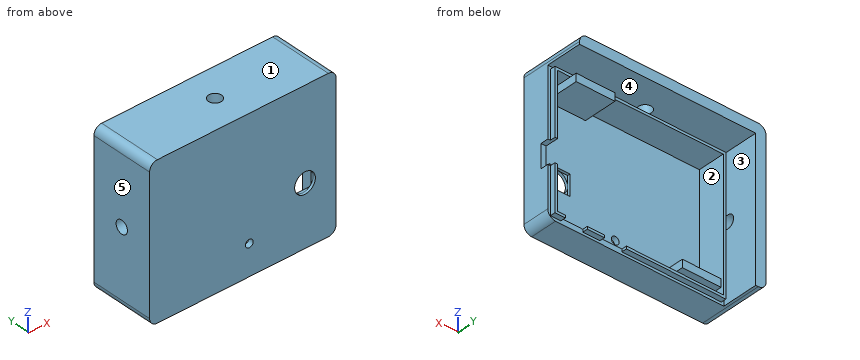
Autodesk Inventor part; units mm, degrees
ref_plane "YZ Plane" through (0, 0, 0) normal (1, 0, 0) x (0, 1, 0)
ref_plane "XZ Plane" through (0, 0, 0) normal (0, 1, 0) x (-1, 0, 0)
ref_plane "XY Plane" through (0, 0, 0) normal (0, 0, 1) x (1, 0, 0)
sketch "Sketch1" plane through (0, 0, 0) normal (0, 1, 0) x (-1, 0, 0)
  point P0 (0, 0)
sketch "Sketch2" plane through (0, 0, 0) normal (0, 1, 0) x (-1, 0, 0)
  line L0 (68, -12) -> (68, -66)
  line L1 (68, -66) -> (0, -66)
  line L2 (0, -66) -> (0, -12)
  line L3 (68, -12) -> (0, -12)
  point P0 (0, 0)
  dimension "d0" = 68
  dimension "d138" = 54
extrude "Extrusion1" add sketch "Sketch2" along normal blind 12.5
sketch "Sketch3" plane through (0, 12.5, 0) normal (0, 1, 0) x (1, 0, 0)
  point P0 (-68, 66)
sketch "Sketch4" plane through (0, 12.5, 0) normal (0, 1, 0) x (1, 0, 0)
  line L0 (0, 66) -> (-68, 66)
  line L1 (-30.4814, 66) -> (-28.4814, 66)
  line L2 (-28.4814, 66) -> (-28.4814, 64)
  line L3 (-68, 66) -> (-68, 12)
  line L4 (-68, 37.8423) -> (-68, 39.8423)
  line L5 (-68, 39.8423) -> (-66, 39.8423)
  line L6 (0, 38.8423) -> (0, 36.8423)
  line L7 (0, 36.8423) -> (-2, 36.8423)
  line L8 (-66, 64) -> (-2, 64)
  line L9 (-2, 64) -> (-2, 14)
  line L10 (-2, 14) -> (-66, 14)
  line L11 (-66, 14) -> (-66, 64)
  dimension "d5" = 2
  dimension "d6" = 2
  dimension "d7" = 2
  dimension "d11" = 2
  dimension "d75" = 2
  dimension "d132" = 50
  dimension "d133" = 64
extrude "Extrusion2" cut sketch "Sketch4" against normal blind 10.5 contours L8 L9 L10 L11
sketch "Sketch7" plane through (0, 12.5, 0) normal (0, 1, 0) x (1, 0, 0)
  line L0 (-68, 66) -> (-67, 66)
  line L1 (-68, 66) -> (-6, 66)
  line L2 (-68, 65) -> (-68, 66)
  line L3 (0, 66) -> (-7, 66)
  line L4 (-67, 65) -> (-1, 65)
  line L5 (0, 66) -> (-68, 66)
  line L6 (-68, 66) -> (0, 66)
  line L7 (0, 12) -> (0, 66)
  line L8 (0, 12) -> (-1, 12)
  line L9 (-1, 66) -> (0, 66)
  line L10 (0, 66) -> (0, 12)
  line L11 (0, 12) -> (-1, 12)
  line L12 (-68, 12) -> (0, 12)
  line L13 (-1, 65) -> (-1, 12)
  line L14 (0, 12) -> (-1, 12)
  line L15 (-67, 65) -> (-67, 12)
  line L16 (-68, 66) -> (-68, 12)
  line L17 (-67, 12) -> (-68, 12)
  line L18 (-68, 12) -> (-68, 66)
  dimension "d76" = 1
  dimension "d139" = 1
  dimension "d140" = 1
extrude "Extrusion3" cut sketch "Sketch7" against normal blind 2 contours L0 L1 L3 L7 L8 L13 L4 L15 L12 L16 L2
sketch "Sketch8" plane through (0, 12.5, 0) normal (0, 1, 0) x (1, 0, 0)
  line L0 (0, 12) -> (0, 13)
  line L1 (0, 13) -> (-68, 13)
  line L2 (0, 12) -> (-68, 12)
  line L3 (-68, 12) -> (-68, 13)
  line L4 (-67, 12) -> (-1, 12)
  point P0 (0, 0)
  point P1 (-70, 0)
  dimension "d46" = 68
  dimension "d141" = 1
extrude "Extrusion4" cut sketch "Sketch8" against normal blind 2
sketch "Sketch10" plane through (0, 2, 0) normal (0, 1, 0) x (1, 0, 0)
  line L0 (-31, 2) -> (-41, 2)
  line L1 (-63, 64) -> (-48, 64)
  line L2 (-48, 64) -> (-48, 61)
  line L3 (-48, 61) -> (-63, 61)
  line L4 (-63, 61) -> (-63, 64)
  line L5 (-22, 14) -> (-7, 14)
  line L6 (-7, 14) -> (-7, 17)
  line L7 (-7, 17) -> (-22, 17)
  line L8 (-22, 17) -> (-22, 14)
  line L9 (-66, 14) -> (-66, 64)
  line L10 (-2, 14) -> (-66, 14)
  line L11 (-66, 64) -> (-2, 64)
  line L12 (-2, 64) -> (-2, 14)
  line L13 (-2, 14) -> (-66, 14)
  line L14 (-66, 14) -> (-66, 64)
  point P0 (0, 0)
  point P1 (-21, 64)
  dimension "d57" = 15
  dimension "d58" = 3
  dimension "d61" = 15
  dimension "d79" = 3
extrude "Extrusion5" add sketch "Sketch10" along normal blind 13 contours L1 L2 L3 L4 | L8 L7 L6 L5
sketch "Sketch11" plane through (0, 0, 0) normal (0, -1, 0) x (1, 0, 0)
  circle A0 centre (-12, -42.73) radius 4
  circle A1 centre (-33.5, -54.23) radius 1.5
  line L0 (0, 0) -> (0, -66)
  line L1 (0, -66) -> (-68, -66)
  line L2 (-2, -64) -> (-2, -14)
  dimension "d85" = 23.27
  dimension "d86" = 21.5
  dimension "d88" = 8
  dimension "d89" = 3
  dimension "d119" = 11.5
  dimension "d120" = 10
extrude "Extrusion6" cut sketch "Sketch11" against normal blind 9
sketch "Sketch12" plane through (0, 0, 0) normal (0, -1, 0) x (1, 0, 0)
  line L0 (-68, -12) -> (-68, -66)
  line L1 (0, -12) -> (0, -8)
  line L2 (0, -8) -> (-68, -8)
  line L3 (-68, -12) -> (0, -12)
  line L4 (0, -12) -> (-68, -12)
  line L5 (-68, -66) -> (-68, -12)
  line L6 (-68, -66) -> (-72, -66)
  line L7 (-68, -12) -> (-68, -66)
  line L8 (-72, -66) -> (-72, -12)
  line L9 (-68, -8) -> (-72, -8)
  line L10 (-72, -8) -> (-72, -12.2471)
  point P0 (0, 0)
  point P1 (-70, 0)
  dimension "d81" = 4
  dimension "d144" = 0
extrude "Extrusion7" add sketch "Sketch12" against normal blind 24.5
sketch "Sketch15" plane through (0, 0, -66) normal (1, 0, 0) x (0, 0, -1)
  line L0 (-27.77, 12.5) -> (-18.77, 12.5)
  line L1 (-18.77, 12.5) -> (-18.77, 7.5)
  line L2 (-18.77, 7.5) -> (-27.77, 7.5)
  line L3 (-27.77, 7.5) -> (-27.77, 12.5)
  line L4 (-54, 0) -> (-54, 24.5)
  line L5 (0, 0) -> (0, 10.5)
  line L6 (0, 0) -> (-58, 0)
  line L7 (0, 10.5) -> (-54, 10.5)
  line L8 (-23.27, -7.8454) -> (-23.27, 0)
  line L9 (-23.27, 0) -> (-23.27, 10.5)
  line L10 (-53, 12.5) -> (-1, 12.5)
  point P0 (-66, 0)
  point P1 (-66, 14.75)
  point P2 (0, 16.75)
  point P3 (-1, 12.5)
  dimension "d108" = 9
  dimension "d109" = 5
  dimension "d111" = 27.77
  dimension "d174" = 0
extrude "Extrusion9" cut sketch "Sketch15" against normal blind 10 contours L0 L1 L7 L3 | L7 L9 L2 L3 | L1 L2 L9 L7
fillet "Fillet7" radius 3 1 edges at (0, 5.25, -66)
fillet "Fillet9" radius 3 1 edges at (0, 12.25, -8)
sketch "Sketch17" plane through (-3, 0, -66) normal (0, 0, -1) x (-1, 0, 0)
  line L0 (2, 15.5) -> (10.5, 15.5)
  line L1 (10.5, 15.5) -> (10.5, 10.5)
  line L2 (10.5, 10.5) -> (2, 10.5)
  line L3 (2, 10.5) -> (2, 15.5)
  line L4 (17.1, 15.5) -> (25.6, 15.5)
  line L5 (25.6, 15.5) -> (25.6, 10.5)
  line L6 (25.6, 10.5) -> (17.1, 10.5)
  line L7 (17.1, 10.5) -> (17.1, 15.5)
  line L8 (66, 0) -> (66, 10.5)
  line L9 (-2, 12.5) -> (64, 12.5)
  line L10 (65, 10.5) -> (0, 10.5)
  line L11 (-3, 10.5) -> (-3, 0)
  point P0 (64, 10.5)
  dimension "d151" = 8.5
  dimension "d152" = 8.5
  dimension "d153" = 5
  dimension "d157" = 0
  dimension "d158" = 13.5
  dimension "d160" = 28.6
extrude "Extrusion11" cut sketch "Sketch17" against normal blind 10 contours L0 L1 L9 L3 | L9 L1 L2 L3 | L9 L5 L6 L7 | L7 L4 L5 L9
sketch "Sketch18" plane through (0, 2, 0) normal (0, 1, 0) x (1, 0, 0)
  circle A0 centre (-12, 42.73) radius 4
  line L0 (-12, 38.73) -> (-8, 38.73)
  line L1 (-8, 38.73) -> (-8, 46.73)
  line L2 (-8, 46.73) -> (-16, 46.73)
  line L3 (-16, 46.73) -> (-16, 38.73)
  line L4 (-16, 38.73) -> (-12, 38.73)
  point P0 (0, 0)
  dimension "d169" = 4
  dimension "d170" = 8
  dimension "d171" = 8
extrude "Extrusion12" cut sketch "Sketch18" against normal blind 1
sketch "Sketch19" plane through (-72, 0, -8) normal (0, 0, 1) x (1, 0, 0)
  line L0 (0, 24.5) -> (69, 24.5)
  line L1 (69, 0) -> (0, 0)
  line L2 (0, 24.5) -> (0, 0)
  line L3 (0, 0) -> (0, 24.5)
  line L4 (0, 12.25) -> (70, 12.25)
  line L5 (4, 10.5) -> (69, 10.5)
  line L6 (72, 10.5) -> (72, 0)
  line L7 (0, 0) -> (72, 0)
  line L8 (0, 4.6147) -> (36, 4.6147)
  line L9 (36, 4.6147) -> (36, 24.5)
  line L10 (72, 24.5) -> (4, 24.5)
  circle A0 centre (36, 12.25) radius 2.5
  dimension "d177" = 36
  dimension "d178" = 5
extrude "Extrusion13" cut sketch "Sketch19" against normal blind 4 contours A0 L9 L4 | L4 L9 L5 A0 | A0 L4 L9 | L4 A0 L5 L9 | L5 L9 A0 | L9 L5 A0
sketch "Sketch20" plane through (-72, 0, -66) normal (-1, 0, 0) x (0, 0, 1)
  line L0 (0, 0) -> (0, 24.5)
  line L1 (0, 12.25) -> (58, 12.25)
  line L2 (58, 24.5) -> (58, 0)
  line L3 (3, 0) -> (55, 0)
  line L4 (29, 0) -> (29, 24.5)
  line L5 (54, 24.5) -> (0, 24.5)
  circle A0 centre (29, 12.25) radius 2.5
  point P0 (66, 0)
  dimension "d181" = 5
extrude "Extrusion14" cut sketch "Sketch20" against normal blind 4 contours A0 L4 L1 | L1 L4 A0 | L4 A0 L1 | L1 A0 L4
fillet "Fillet12" radius 3 1 edges at (-72, 12.25, -8)
fillet "Fillet13" radius 3 1 edges at (-72, 12.25, -66)
properties part number "Shell 4 top"
Model file for the job. Use its own axes, mm. Face numbers are marked on the shaded views. A direction names the side the tool comes from. Round coordinates to 2 decimals unless told otherwise and drop trailing zeros. Loops run counter-clockwise (first coordinate to the right, second up) from the corner with the lowest first, then second, coordinate; pieces in that order, holes last. Notation, with made-up numbers: M 30,87.25 L 36,87.25 A14 cw 36,102.25 Z; hole C 74,13 d2. An arc over 180 degrees is marked long. Put each result on its own line as item: value. Start each with the question number.
Item 1: 3-axis set-ups, long thin cutter, end or side, ignore diameter. For the marked faces 1 and 2: which of +Z, -Z, +X, -X, +Y, -Y reach the whole face in a straight line?
Item 2: Cut at D-D (x = -37). List the corners of the cut face in (y, z).
Item 3: Mould opens along X. For the marked faces 3, 4 and 5 say: released by +X, released by -X, zero draft, split by the parting line, or undercut.
Item 4: Drop flat-ended pins along their axis: P1, Ø2.5, axis at x = -33.5, z = -54.23, coming from the +Y side; P2, Ø1, axis at x = -23, z = -20, coming from the +Y side; P3, Ø1.1, axis at y = 11.5, z = -64.5, coming from the -X side; P4, Ø1.5, axis at x = -17.5, z = -15.5, coming from the +Y side. Give the stop position or say it passes through.
Item 5: Cut at B-B (x = -26). List the corners of the cut face in (y, z), then the cut area to 3 significant figures.
Item 6: Drill centre lines: line 1 along Y through (x, z) = (-36, -9.75); line 2 along X through (y, z) = (10, -27); line 3 along Z through (x, y) = (-12, 0.4). Where is each one in solid material? Low to high.
Item 7: Cut at C-C (y = 18.75). List the corners of the cut face in (x, z), then the cut area to 3 significant figures.
Item 8: Cut at A-A (z = -54.23). List the corners of the cut face in (x, y), then the cut area to 3 significant figures.
Answer block:
1. face 1: +Z, +X, -X, +Y, -Y
1. face 2: +Y
2. outline: M 0,-66 L 10.5,-66 L 10.5,-65 L 12.5,-65 L 12.5,-64 L 2,-64 L 2,-14 L 12.5,-14 L 12.5,-13 L 10.5,-13 L 10.5,-12 L 9.96,-12 L 9.96,-8 L 0,-8 Z; M 14.54,-12 L 24.5,-12 L 24.5,-8 L 14.54,-8 Z
3. face 3: undercut
3. face 4: zero draft
3. face 5: released by -X
4. P1: through
4. P2: y = 2
4. P3: x = -71.85
4. P4: y = 15
5. outline: M 0,-66 L 10.5,-66 L 10.5,-64 L 2,-64 L 2,-14 L 12.5,-14 L 12.5,-13 L 10.5,-13 L 10.5,-12 L 24.5,-12 L 24.5,-8 L 0,-8 Z
5. area: 242 mm2
6. line 1: 0 to 9.75, 14.75 to 24.5
6. line 2: -72 to -66, -2 to 0
6. line 3: -66 to -46.73, -38.73 to -8
7. outline: M -72,-63 A3 ccw -69,-66 L -68,-66 L -68,-12 L 0,-12 L 0,-11 A3 ccw -3,-8 L -69,-8 A3 ccw -72,-11 Z
7. area: 498 mm2
8. outline: M -72,0 L -35,0 L -35,2 L -66,2 L -66,12.5 L -67,12.5 L -67,10.5 L -68,10.5 L -68,24.5 L -72,24.5 Z; M -32,0 L 0,0 L 0,10.5 L -1,10.5 L -1,12.5 L -2,12.5 L -2,2 L -32,2 Z
8. area: 266 mm2
